```python
from build123d import *

# Parameters (mm, degrees)
F0_W          = 50
F0_H          = 50
F1_DEPTH      = 5
F2_R          = 3.25
F3_DEPTH      = 8
F3_DEPTH_BACK = 3
F4_R          = 3.25
F5_DEPTH      = 3
F5_DEPTH_BACK = 3
F6_T4_DEPTH   = 60
F6_S5_R       = 3.25
F6_T6_DEPTH   = 32
F6_T10_DEPTH  = 60


# Not quite as in the source:
# - a fillet or chamfer that OpenCascade refuses, or shapes differently, is made with other operations: its cross-section is extruded or revolved along the edge and cut away or added


with BuildPart() as f1:
    # F0 (on Front) → F1 (new body)
    with BuildSketch(Plane.XZ):
        with Locations((25, 25)):
            Rectangle(F0_W, F0_H)
    extrude(amount=F1_DEPTH)

    # F2 (on face) → F3 (join, two sides)
    with BuildSketch(Plane(origin=(0, 0, 0), x_dir=(1, 0, 0), z_dir=(0, 0, -1))) as f3_sk:
        with Locations((3, 3)):
            Circle(F2_R)
    extrude(amount=F3_DEPTH)
    extrude(f3_sk.sketch, amount=-F3_DEPTH_BACK)

    # F4 (on face) → F5 (join, two sides)
    with BuildSketch(Plane.XY.offset(50)) as f5_sk:
        with Locations((3, -3)):
            Circle(F4_R)
    extrude(amount=F5_DEPTH)
    extrude(f5_sk.sketch, amount=-F5_DEPTH_BACK)

    # F6: fillet of radius 2 on 1 edges, made by hand


with BuildPart() as f6_tool2:
    # F6_s3 → F6_t4 (new body)
    with BuildSketch(Plane.XY.offset(55)):
        with BuildLine():
            ThreePointArc((0, -2), (0.5857864376, -0.5857864376), (2, 0))
            Line((2, 0), (0, 0))
            Line((0, 0), (0, -2))
        make_face()
    extrude(amount=-F6_T4_DEPTH)

    # F6_s5 → F6_t6 (cut, symmetric)
    with BuildSketch(Plane.XY.offset(25)):
        with Locations((3, -3)):
            Circle(F6_S5_R)
    extrude(amount=F6_T6_DEPTH, both=True, mode=Mode.SUBTRACT)


with BuildPart() as f1_1:
    add(f1.part)

    # F6_t1: cut F6_tool2
    add(f6_tool2.part, mode=Mode.SUBTRACT)


with BuildPart() as f6_tool8:
    # F6_s9 → F6_t10 (new body)
    with BuildSketch(Plane.XY.offset(55)):
        with BuildLine():
            ThreePointArc((0, -2), (0.5857864376, -0.5857864376), (2, 0))
            Line((2, 0), (0, 0))
            Line((0, 0), (0, -2))
        make_face()
    extrude(amount=-F6_T10_DEPTH)

    split(bisect_by=Plane.XY.offset(3), keep=Keep.TOP)

    split(bisect_by=Plane.XY.offset(47), keep=Keep.BOTTOM)


with BuildPart() as f1_2:
    add(f1_1.part)

    # F6_t7: cut F6_tool8
    add(f6_tool8.part, mode=Mode.SUBTRACT)


solid = f1_2.part
```
Model file for the job. Use its own axes, mm. A direction names the side the tool comes from. Coordinates: 2 decimals unless noted, no trailing zeros. Write each loop counter-clockwise with the first axis right and the second up, starting at its lowest first coordinate (ties: lowest second). Pieces come first, ordered by that corner, then holes. Notation, with made-up numbers: (-16.75, -10) - (-5.75, -10) arc R18 cw to (-5.75, 25) - close; hole circle Ø8 at (-11, -26). An arc over 180 degrees is marked (long way). One line per item, written item: value. Start each with the question number.
1. Tool access for faces 1 (the flat face through (50, -2, 25)), 2 (the flat face through (3, -5.5, 47)): list every direction of +Z, -Z, +X, -X, +Y, -Y with a clear straight run to the whole face (end or side of a thin tool).
2. Slice it at B-B (z = 6). Write the cut outline in (x, y).
3. Probe line 1 (Z direction, x = 4, y = -6); line 2 (Z direction, x = 44, y = -4.5); line 3 (Y direction, x = 38, z = 7). List the from-to ranges inside material, lowest first. Write a range as from..to.
4. Flat gauge pins, fed straight in: pin 1 (1.5 mm diameter, centred on x = 35.5, y = -4, fed in from +Z); pin 2 (1 mm diameter, centred on x = 25.5, z = 40, fed in from +Y); pin 3 (2.5 mm diameter, centred on y = -4, z = 25, fed in from -X). Where does each tip first touch, or does it go through?
5. Slice it at A-A (x = 3). Write the cut outline in (y, z), plus the area to 4 significant figures.
6. Mould opens along Z. For faces 3 (the flat face through (27, -2, 50)), 4 (the flat face through (27, -2, 0)), 5 (the flat face through (3, -5.5, 3)) say: released by +Z, released by -Z, zero draft, split by the parting line, or undercut.
7. Slice it at C-C (z = -3.5). Write the cut outline in (x, y), plus the area to 3 significant figures.
Answers below:
1. face 1: +Z, -Z, +X, +Y, -Y
1. face 2: +X, -X, -Y
2. outline: (0, -5) - (50, -5) - (50, 0) - (2, 0) arc R2 ccw to (0, -2) - close
3. line 1: z = -8..3, 47..53
3. line 2: z = 0..50
3. line 3: y = -5..0
4. pin 1: stops at z = 50
4. pin 2: stops at y = 0
4. pin 3: stops at x = 0
5. outline: (-6.25, -8) - (0.25, -8) - (0.25, 3) - (0, 3) - (0, 47) - (0.25, 47) - (0.25, 53) - (-6.25, 53) - (-6.25, 47) - (-5, 47) - (-5, 3) - (-6.25, 3) - close
5. area: 330.5 mm^2
6. face 3: released by +Z
6. face 4: released by -Z
6. face 5: undercut
7. outline: circle Ø6.5 at (3, -3)
7. area: 33.2 mm^2
